Source: three-view drawing plus pictorial views. Frame: mm from the lowest corner of the part. A direction names the side the tool comes from. Coordinates: 2 decimals unless noted, no trailing zeros. Order: outer loops, then holes, each group sorted by start corner. A loop starts at its lowest first (then second) coordinate and runs counter-clockwise, first axis right, second up. Notation, with made-up numbers: M -29.5,-37 L 13.5,-37 A30 ccw 13.5,-4 Z; hole C 61,-22.5 d11. An arc over 180 degrees is marked long. One line per question, with ' | ' between items.
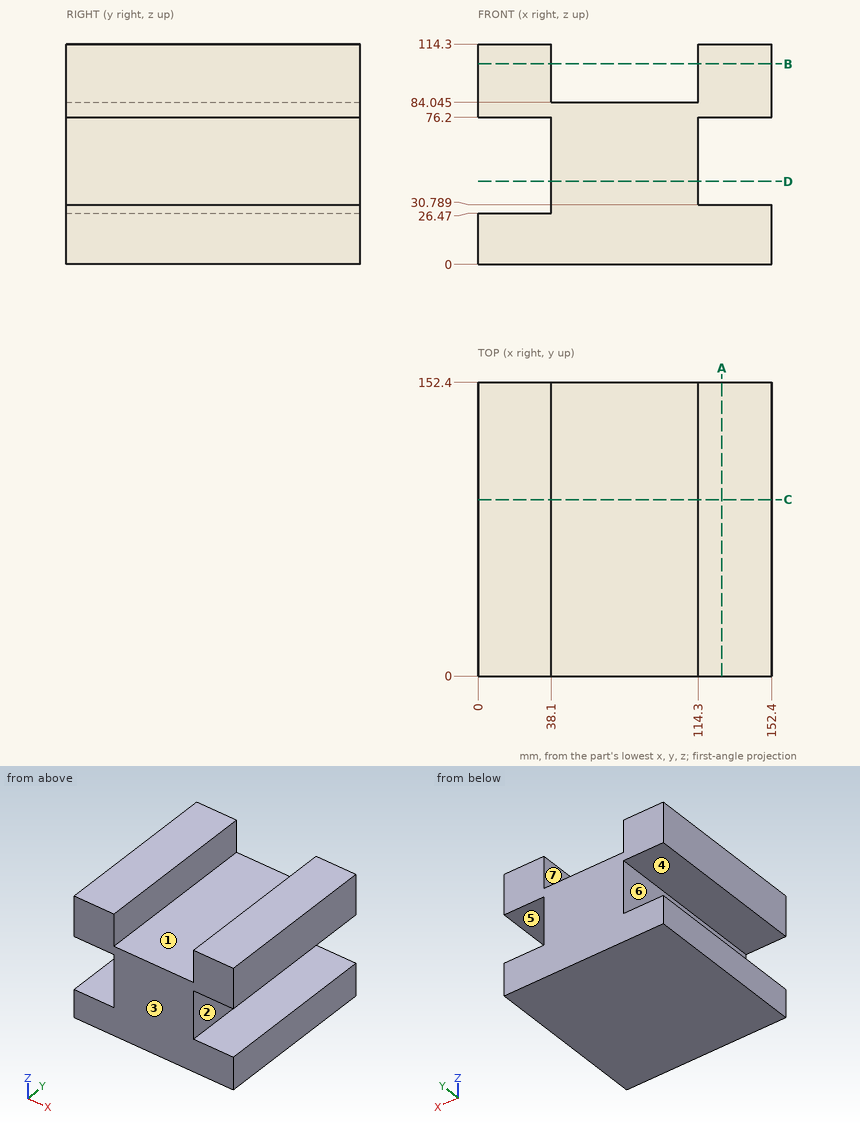
1. Material intervals for line 1 (X direction, y = 89, z = 95.5); line 2 (Z direction, x = 131.5, y = 134); line 3 (Z direction, x = 33, y = 99), sorted ascending. Write a range as [from, to].
Response values:
line 1: x = [0, 38.1], [114.3, 152.4] | line 2: z = [0, 30.79], [76.2, 114.3] | line 3: z = [0, 26.47], [76.2, 114.3]
2. Draft query along X for the marked faces 5, 6 and 7. Return one class per face: pulls with the +X half, pulls with the -X half, needs draft (parallel to the pull), parting line crosses it, or undercut.
Response values:
face 5: needs draft | face 6: pulls with the -X half | face 7: undercut
3. Section C-C, the plane y = 91.5. Output: boundary loops of the cut face in (x, z) (1 decimal), and give its area (3 significant figures).
Response values:
outline: M 0,0 L 152.4,0 L 152.4,30.8 L 114.3,30.8 L 114.3,76.2 L 152.4,76.2 L 152.4,114.3 L 114.3,114.3 L 114.3,84 L 38.1,84 L 38.1,114.3 L 0,114.3 L 0,76.2 L 38.1,76.2 L 38.1,26.5 L 0,26.5 Z | area: 11,500 mm^2
4. Section A-A, the plane x = 126.5. Output: boundary loops of the cut face in (y, z), and give its area (3 significant figures).
Response values:
outline: M 0,0 L 152.4,0 L 152.4,30.79 L 0,30.79 Z; M 0,76.2 L 152.4,76.2 L 152.4,114.3 L 0,114.3 Z | area: 10,500 mm^2
5. Section D-D, the plane z = 43. Output: boundary loops of the cut face in (x, y), and give its area (3 significant figures).
Response values:
outline: M 38.1,0 L 114.3,0 L 114.3,152.4 L 38.1,152.4 Z | area: 11,600 mm^2
6. Pin query (flat end, axial travel): P1, Ø22.5, axis at y = 55, z = 43, coming from the +X side; P2, Ø3, axis at x = 135.5, z = 12.5, coming from the -Y side; P3, Ø25, axis at y = 88.5, z = 46, coming from the -X side; P4, Ø23, axis at x = 80.5, y = 56, coming from the +Z side (1 decimal). Return the tip coordinate at first contact, or that it passes through.
Response values:
P1: stops at x = 114.3 | P2: stops at y = 0 | P3: stops at x = 38.1 | P4: stops at z = 84
7. Section B-B, the plane z = 104. Output: boundary loops of the cut face in (x, y).
Response values:
outline: M 0,0 L 38.1,0 L 38.1,152.4 L 0,152.4 Z; M 114.3,0 L 152.4,0 L 152.4,152.4 L 114.3,152.4 Z
8. Access query for the marked faces 1, 2, 3 and 4. Directions: +Z, -Z, +X, -X, +Y, -Y. A direction counts if a zero-diameter tool reaches every point of the face in a straight line with its end or side. Return the directions, or none.
Response values:
face 1: +Z, +Y, -Y | face 2: +X, +Y, -Y | face 3: +Z, -Z, +X, -X, -Y | face 4: -X, +Y, -Y
